The model under review builds one solid part; all positions refer to its coordinate system, in mm. Round coordinates to 2 decimals unless told otherwise and drop trailing zeros. Order: outer loops, then holes, each group sorted by start corner. A loop starts at its lowest first (then second) coordinate and runs counter-clockwise, first axis right, second up.
```python
from build123d import *

# Parameters (mm, degrees)
SKETCH1_W           = 96
SKETCH1_H           = 58.35
SKETCH1_R           = 2.05
SKETCH1_W_2         = 17
SKETCH1_H_2         = 36
BOSS_EXTRUDE1_DEPTH = 3.175
FILLET1_R           = 4


with BuildPart() as part:
    # Sketch1 → Boss-Extrude1 (new body)
    with BuildSketch(Plane.XY):
        Rectangle(SKETCH1_W, SKETCH1_H)
        with Locations((-42.5, 18)):
            Circle(SKETCH1_R, mode=Mode.SUBTRACT)
        with Locations((-42.5, -18)):
            Circle(SKETCH1_R, mode=Mode.SUBTRACT)
        with Locations((42.5, 18)):
            Circle(SKETCH1_R, mode=Mode.SUBTRACT)
        with Locations((42.5, -18)):
            Circle(SKETCH1_R, mode=Mode.SUBTRACT)
        with Locations((8, -8)):
            Circle(SKETCH1_R, mode=Mode.SUBTRACT)
        with Locations((-8, -8)):
            Circle(SKETCH1_R, mode=Mode.SUBTRACT)
        with Locations((-8, 8)):
            Circle(SKETCH1_R, mode=Mode.SUBTRACT)
        with Locations((8, 8)):
            Circle(SKETCH1_R, mode=Mode.SUBTRACT)
        with Locations((-30, 0)):
            Rectangle(SKETCH1_W_2, SKETCH1_H_2, mode=Mode.SUBTRACT)
        with Locations((30, 0)):
            Rectangle(SKETCH1_W_2, SKETCH1_H_2, mode=Mode.SUBTRACT)
    extrude(amount=BOSS_EXTRUDE1_DEPTH)

    # Fillet1
    fillet1_edges = [part.edges().sort_by_distance(p)[0] for p in [
        (-21.5, 18, 1.5875),
        (-38.5, 18, 1.5875),
        (-38.5, -18, 1.5875),
        (-21.5, -18, 1.5875),
        (21.5, -18, 1.5875),
        (38.5, -18, 1.5875),
        (38.5, 18, 1.5875),
        (21.5, 18, 1.5875),
        (-48, 29.175, 1.5875),
        (48, 29.175, 1.5875),
        (48, -29.175, 1.5875),
        (-48, -29.175, 1.5875),
    ]]
    fillet(fillet1_edges, radius=FILLET1_R)


solid = part.part
```
(1) Consider section C-C (z = 0.9). State how many separate pieces and enclosed holes the cut face has, and give its area (3 significant figures).
Data:
separate pieces: 1
enclosed holes: 10
area: 4,290 mm2
(2) Consider section B-B (y = 8). Write out the cut boundary in (x, z) (3 decimals).
Data:
outline: (-48, 0) - (-38.5, 0) - (-38.5, 3.175) - (-48, 3.175) - close; (-21.5, 0) - (-10.05, 0) - (-10.05, 3.175) - (-21.5, 3.175) - close; (-5.95, 0) - (5.95, 0) - (5.95, 3.175) - (-5.95, 3.175) - close; (10.05, 0) - (21.5, 0) - (21.5, 3.175) - (10.05, 3.175) - close; (38.5, 0) - (48, 0) - (48, 3.175) - (38.5, 3.175) - close
(3) Draft analysis for pull direction Y (two halves, no side actions). For faces 1 (the flat face through (-48, 0, 2)), 2 (the flat face through (21.5, 0, 2)), 3 (the cylindrical face through (-22.703, -16.859, 1.61)), 4 (the flat face through (-1, 29.175, 2)), state which applies: pulls with the +Y half, pulls with the -Y half, needs draft (parallel to the pull), parting line crosses it, or undercut.
Data:
face 1: needs draft
face 2: undercut
face 3: undercut
face 4: pulls with the +Y half
(4) To check wall thickness, follow probe 1 along Y at (x, z) = (-8, 2.5) (3 decimals); probe 2 along X at (y, z) = (3.5, 0.3); probe 3 along X at (y, z) = (15.5, 2.25). State the ranges of each line that lie inside material, in increasing order.
Data:
probe 1: y = -29.175 to -10.05, -5.95 to 5.95, 10.05 to 29.175
probe 2: x = -48 to -38.5, -21.5 to 21.5, 38.5 to 48
probe 3: x = -48 to -38.21, -21.79 to 21.79, 38.21 to 48
(5) Consider section A-A (x = -8). Write out the cut boundary in (y, z) (3 decimals), and give its area (3 significant figures).
Data:
outline: (-29.175, 0) - (-10.05, 0) - (-10.05, 3.175) - (-29.175, 3.175) - close; (-5.95, 0) - (5.95, 0) - (5.95, 3.175) - (-5.95, 3.175) - close; (10.05, 0) - (29.175, 0) - (29.175, 3.175) - (10.05, 3.175) - close
area: 159 mm2
(6) Consider section D-D (y = 19). Write out the cut boundary in (x, z) (3 decimals), and give its area (3 significant figures).
Data:
outline: (-48, 0) - (-44.29, 0) - (-44.29, 3.175) - (-48, 3.175) - close; (-40.71, 0) - (40.71, 0) - (40.71, 3.175) - (-40.71, 3.175) - close; (44.29, 0) - (48, 0) - (48, 3.175) - (44.29, 3.175) - close
area: 282 mm2
